```python
from build123d import *

# Parameters (mm, degrees)
SKETCH_1_W          = 140
SKETCH_1_H          = 90
EXTRUDE_1_DEPTH     = 5
SKETCH_2_W          = 5
SKETCH_2_H          = 90
EXTRUDE_2_DEPTH     = 9
SKETCH_3_R          = 1.75
CUT_EXTRUDE_1_DEPTH = 11
SKETCH_5_W          = 30.6
SKETCH_5_H          = 10.6
SKETCH_5_R          = 1.75
CUT_EXTRUDE_2_DEPTH = 2
SKETCH_5_3_R        = 1.75
CUT_EXTRUDE_3_DEPTH = 6
FILLET_1_R          = 2
FILLET_2_R          = 1


with BuildPart() as part:
    # Sketch 1 → Extrude 1 (new body)
    with BuildSketch(Plane(origin=(0, 0, 0), x_dir=(1, 0, 0), z_dir=(0, 1, 0))):
        Rectangle(SKETCH_1_W, SKETCH_1_H)
    extrude(amount=EXTRUDE_1_DEPTH)

    # Sketch 2 → Extrude 2 (add)
    with BuildSketch(Plane(origin=(0, 5, 0), x_dir=(1, 0, 0), z_dir=(0, 1, 0))):
        with Locations((-67.5, 0)):
            Rectangle(SKETCH_2_W, SKETCH_2_H)
    extrude(amount=EXTRUDE_2_DEPTH)

    # Sketch 3 → Cut-Extrude 1 (cut)
    with BuildSketch(Plane.ZY.offset(70)):
        with Locations((30, 9)):
            Circle(SKETCH_3_R)
        with Locations((10, 9)):
            Circle(SKETCH_3_R)
        with Locations((-10, 9)):
            Circle(SKETCH_3_R)
        with Locations((-30, 9)):
            Circle(SKETCH_3_R)
    extrude(amount=-CUT_EXTRUDE_1_DEPTH, mode=Mode.SUBTRACT)

    # Sketch 5 → Cut-Extrude 2 (cut)
    with BuildSketch(Plane(origin=(0, 5, 0), x_dir=(1, 0, 0), z_dir=(0, 1, 0))):
        with Locations((-35.3, -19.7)):
            Rectangle(SKETCH_5_W, SKETCH_5_H)
        with Locations((-46.8, -19.7)):
            Circle(SKETCH_5_R, mode=Mode.SUBTRACT)
        with Locations((-23.8, -19.7)):
            Circle(SKETCH_5_R, mode=Mode.SUBTRACT)
        with Locations((-35.3, 19.7)):
            Rectangle(SKETCH_5_W, SKETCH_5_H)
        with Locations((-23.8, 19.7)):
            Circle(SKETCH_5_R, mode=Mode.SUBTRACT)
        with Locations((-46.8, 19.7)):
            Circle(SKETCH_5_R, mode=Mode.SUBTRACT)
        with Locations((35.3, 19.7)):
            Rectangle(SKETCH_5_W, SKETCH_5_H)
        with Locations((46.8, 19.7)):
            Circle(SKETCH_5_R, mode=Mode.SUBTRACT)
        with Locations((23.8, 19.7)):
            Circle(SKETCH_5_R, mode=Mode.SUBTRACT)
        with Locations((35.3, -19.7)):
            Rectangle(SKETCH_5_W, SKETCH_5_H)
        with Locations((23.8, -19.7)):
            Circle(SKETCH_5_R, mode=Mode.SUBTRACT)
        with Locations((46.8, -19.7)):
            Circle(SKETCH_5_R, mode=Mode.SUBTRACT)
    extrude(amount=-CUT_EXTRUDE_2_DEPTH, mode=Mode.SUBTRACT)

    # Sketch 5_3 → Cut-Extrude 3 (cut, through all)
    with BuildSketch(Plane(origin=(0, 5, 0), x_dir=(1, 0, 0), z_dir=(0, 1, 0))):
        with Locations((46.8, -19.7)):
            Circle(SKETCH_5_3_R)
        with Locations((23.8, -19.7)):
            Circle(SKETCH_5_3_R)
        with Locations((46.8, 19.7)):
            Circle(SKETCH_5_3_R)
        with Locations((23.8, 19.7)):
            Circle(SKETCH_5_3_R)
        with Locations((-23.8, 19.7)):
            Circle(SKETCH_5_3_R)
        with Locations((-23.8, -19.7)):
            Circle(SKETCH_5_3_R)
        with Locations((-46.8, -19.7)):
            Circle(SKETCH_5_3_R)
        with Locations((-46.8, 19.7)):
            Circle(SKETCH_5_3_R)
    extrude(amount=-CUT_EXTRUDE_3_DEPTH, mode=Mode.SUBTRACT)

    # Fillet 1
    fillet_1_edges = [part.edges().sort_by_distance(p)[0] for p in [
        (70, 0, 0),
        (70, 5, 0),
        (-65, 14, 0),
        (-70, 14, 0),
        (-70, 0, 0),
        (0, 0, -45),
        (2.5, 5, -45),
        (0, 0, 45),
        (2.5, 5, 45),
        (-65, 9.5, 45),
        (-65, 9.5, -45),
        (-70, 7, 45),
        (-70, 7, -45),
        (70, 2.5, 45),
        (70, 2.5, -45),
    ]]
    fillet(fillet_1_edges, radius=FILLET_1_R)

    # Fillet 2
    fillet_2_edges = [part.edges().sort_by_distance(p)[0] for p in [
        (35.3, 5, 25),
        (50.6, 5, 19.7),
        (35.3, 5, 14.4),
        (20, 5, 19.7),
        (-20, 5, 19.7),
        (-35.3, 5, 14.4),
        (-50.6, 5, 19.7),
        (-35.3, 5, 25),
        (-35.3, 5, -25),
        (-50.6, 5, -19.7),
        (-35.3, 5, -14.4),
        (-20, 5, -19.7),
        (20, 5, -19.7),
        (35.3, 5, -14.4),
        (50.6, 5, -19.7),
        (35.3, 5, -25),
    ]]
    fillet(fillet_2_edges, radius=FILLET_2_R)


solid = part.part
```
For this review, take the finished solid that the model builds, in its own axes (mm). A direction names the side the tool comes from. Give positions to 0.01 mm unless a question says otherwise; leave off trailing zeros. Write each loop counter-clockwise with the first axis right and the second up, starting at its lowest first coordinate (ties: lowest second). Pieces come first, ordered by that corner, then holes.
Item 1: Take a section at D-D (z = 19.7). Give the number of separate pieces and of enclosed holes in the cut face, and give its area (3 significant figures).
Item 2: Take a section at C-C (z = 30). Give the boundary of the cut face in (x, y), and give its area (3 significant figures).
Item 3: The part is to be moulded in two halves that separate along Z. For faces 1 (the face through (-70, 7, 1)), 2 (the face through (-0.3, 2.2, -45)), 3 (the face through (-67.5, 10.5, 10.9)), say which applies: +Z half, -Z half, draft (parallel to the pull), parting line (faces both ways), or undercut.
Item 4: Machinability: for faces 4 (the face through (-67.54, 9.08, -31.75)), 5 (the face through (35, 3, -20)), 6 (the face through (-65, 8, 1)), which of the approach directions +Z, -Z, +X, -X, +Y, -Y give a long, thin tool a straight path to every point of the face, cutting with its end or side? Answer none if there is none.
Item 5: Take a section at A-A (x = 23.8). Give the boundary of the cut face in (y, z), and give its area (3 significant figures).
Item 6: Wall thickness on probe 1 along X at (y, z) = (2.25, 19.7); probe 2 along Z at (x, y) = (46.8, 1.8); probe 3 along Z at (x, y) = (46.8, 0.6): over which ranges is each line inside the solid? List them lowest first.
Item 7: Insertion check: P1, Ø3.5, axis at y = 9, z = 11, coming from the +X side; P2, Ø11.5, axis at x = -41, z = -17, coming from the +Y side; P3, Ø0.5, axis at x = 32, y = 3.5, coming from the +Z side. Each pin has a flat end and moves straight along its axis. Give the tip position at first contact, or say it passes through.
Item 8: Take a section at B-B (y = 9). Give the boundary of the cut face in (x, z), and give its area (3 significant figures).
Established:
1. separate pieces: 5
1. enclosed holes: 0
1. area: 575 mm2
2. outline: (-70, 2) arc R2 ccw to (-68, 0) - (68, 0) arc R2 ccw to (70, 2) - (70, 3) arc R2 ccw to (68, 5) - (-65, 5) - (-65, 7.25) - (-70, 7.25) - close; (-70, 10.75) - (-65, 10.75) - (-65, 12) arc R2 ccw to (-67, 14) - (-68, 14) arc R2 ccw to (-70, 12) - close
2. area: 723 mm2
3. face 1: draft
3. face 2: -Z half
3. face 3: undercut
4. face 4: +X, -X
4. face 5: +Y
4. face 6: +Z, -Z, +X, +Y
5. outline: (0, -43) arc R2 ccw to (2, -45) - (3, -45) arc R2 ccw to (5, -43) - (5, -26) arc R1 ccw to (4, -25) - (3, -25) - (3, -21.45) - (0, -21.45) - close; (0, -17.95) - (3, -17.95) - (3, -14.4) - (4, -14.4) arc R1 ccw to (5, -13.4) - (5, 13.4) arc R1 ccw to (4, 14.4) - (3, 14.4) - (3, 17.95) - (0, 17.95) - close; (0, 21.45) - (3, 21.45) - (3, 25) - (4, 25) arc R1 ccw to (5, 26) - (5, 43) arc R2 ccw to (3, 45) - (2, 45) arc R2 ccw to (0, 43) - close
5. area: 382 mm2
6. probe 1: x = -70 to -48.55, -45.05 to -25.55, -22.05 to 22.05, 25.55 to 45.05, 48.55 to 70
6. probe 2: z = -44.99 to -21.45, -17.95 to 17.95, 21.45 to 44.99
6. probe 3: z = -44.43 to -21.45, -17.95 to 17.95, 21.45 to 44.43
7. P1: stops at x = -65
7. P2: stops at y = 5
7. P3: stops at z = 44.98
8. outline: (-70, -43) arc R2 ccw to (-68, -45) - (-67, -45) arc R2 ccw to (-65, -43) - (-65, -31.75) - (-70, -31.75) - close; (-70, -28.25) - (-65, -28.25) - (-65, -11.75) - (-70, -11.75) - close; (-70, -8.25) - (-65, -8.25) - (-65, 8.25) - (-70, 8.25) - close; (-70, 11.75) - (-65, 11.75) - (-65, 28.25) - (-70, 28.25) - close; (-70, 31.75) - (-65, 31.75) - (-65, 43) arc R2 ccw to (-67, 45) - (-68, 45) arc R2 ccw to (-70, 43) - close
8. area: 377 mm2
